Work out the finished part from the listing and answer in its coordinate system (mm). A direction names the side the tool comes from. Coordinates: 2 decimals unless noted, no trailing zeros. Order: outer loops, then holes, each group sorted by start corner. A loop starts at its lowest first (then second) coordinate and runs counter-clockwise, first axis right, second up.
1. The part is cut by section C-C, the plane z = -66. Give the vertices of the cut face in (x, y).
2. Determine the mould class of faces 1 (the flat face through (0.6, -5, -39.8)), 2 (the flat face through (3.133, -3.854, -71.022)) for opening direction Z: +Z half, -Z half, draft (parallel to the pull), parting line (faces both ways), or undercut.
3. The part is cut by section B-B, the plane y = -1.2. Give the vertices of the cut face in (x, z), then the cut area to 3 significant figures.
4. Find the intervals of material crossed by probe 1 along Z at (x, y) = (0, -2.9); probe 2 along X at (y, z) = (-1.6, -16); probe 3 along X at (y, z) = (-2.95, -32), in increasing order.
5. A tool of negligible diameter and unlimited length cuts with its end or side. For faces 3 (the flat face through (3, -2, -40)), 4 (the flat face through (5.61, -2.47, -6.72)), 5 (the flat face through (-4, -1, -40)), 6 (the flat face through (-3.17, -3.48, -10.05)), from which of +Z, -Z, +X, -X, +Y, -Y can it reach the whole face along a straight path? Write none if from no direction.
6. The part is cut by section A-A, the plane z = -55.5. Give the vertices of the cut face in (x, y), then the cut area to 3 significant figures.
7. Flat-ended cylindrical pins translate along their axes: pin 1 Ø0.9 at (y, z) = (-3, -27.5) entering from +X; pin 2 Ø2 at (y, z) = (-3, -68.5) entering from +X; pin 3 Ø1.5 at (y, z) = (-4.5, -25.5) entering from -X. Find the tip coordinate at first contact, or state that the pin passes through.
```python
from build123d import *

# Parameters (mm, degrees)
F0_W      = 4
F0_H      = 5.1029750705
F1_DEPTH  = 5
F4_DEPTH  = 9
F6_W      = 44.082082808
F6_H      = 137.8899626434
F7_DEPTH  = 25
F9_R      = 1.5
F10_DEPTH = 25


with BuildPart() as f1:
    # F0 (on Front) → F1 (new body)
    with BuildSketch(Plane.XZ):
        with Locations((2, -12.5514875352)):
            Rectangle(F0_W, F0_H)
        with BuildLine():
            Line((-4, -10), (0, -10))
            Line((0, -10), (0, -8))
            ThreePointArc((0, -8), (-2.0705523608, -7.7274066103), (-4, -6.9282032303))
            Line((-4, -6.9282032303), (-4, -10))
        make_face()
        with Locations((-2, -12.5514875352)):
            Rectangle(F0_W, F0_H)
        with BuildLine():
            Line((0, -8), (0, -10))
            Line((0, -10), (4, -10))
            Line((4, -10), (4, -6.9282032303))
            ThreePointArc((4, -6.9282032303), (2.0705523608, -7.7274066103), (0, -8))
        make_face()
        with BuildLine():
            Line((4, -15.1029750705), (0, -15.1029750705))
            Line((0, -15.1029750705), (0, -65))
            Line((0, -65), (0, -70))
            Line((0, -70), (0, -72))
            ThreePointArc((0, -72), (2.0705523608, -72.2725933897), (4, -73.0717967697))
            Line((4, -73.0717967697), (4, -70))
            Line((4, -70), (4, -15.1029750705))
        make_face()
        with BuildLine():
            Line((0, -65), (0, -15.1029750705))
            Line((0, -15.1029750705), (-4, -15.1029750705))
            Line((-4, -15.1029750705), (-4, -70))
            Line((-4, -70), (-4, -73.0717967697))
            ThreePointArc((-4, -73.0717967697), (-2.0705523608, -72.2725933897), (0, -72))
            Line((0, -72), (0, -70))
            Line((0, -70), (0, -65))
        make_face()
        with BuildLine():
            ThreePointArc((-4, -6.9282032303), (-2.0705523608, -7.7274066103), (0, -8))
            ThreePointArc((0, -8), (2.0705523608, -7.7274066103), (4, -6.9282032303))
            ThreePointArc((4, -6.9282032303), (5.8428493863, -5.4645320979), (7.1800707248, -3.5279717101))
            ThreePointArc((7.1800707248, -3.5279717101), (7.792322048, -1.8109989235), (8, 0))
            ThreePointArc((8, 0), (-1.8109989235, 7.792322048), (-7.1800707248, -3.5279717101))
            ThreePointArc((-7.1800707248, -3.5279717101), (-5.8428493863, -5.4645320979), (-4, -6.9282032303))
        make_face()
        with BuildLine():
            Line((-7.1800707248, -3.5279717101), (-4, -10))
            Line((-4, -10), (-4, -6.9282032303))
            ThreePointArc((-4, -6.9282032303), (-5.8428493863, -5.4645320979), (-7.1800707248, -3.5279717101))
        make_face()
        with BuildLine():
            Line((4, -6.9282032303), (4, -10))
            Line((4, -10), (7.1800707248, -3.5279717101))
            ThreePointArc((7.1800707248, -3.5279717101), (5.8428493863, -5.4645320979), (4, -6.9282032303))
        make_face()
        with BuildLine():
            Line((-4, -73.0717967697), (-4, -70))
            Line((-4, -70), (-7.1800707248, -76.4720282899))
            ThreePointArc((-7.1800707248, -76.4720282899), (-5.8428493863, -74.5354679021), (-4, -73.0717967697))
        make_face()
        with BuildLine():
            Line((7.1800707248, -76.4720282899), (4, -70))
            Line((4, -70), (4, -73.0717967697))
            ThreePointArc((4, -73.0717967697), (5.8428493863, -74.5354679021), (7.1800707248, -76.4720282899))
        make_face()
        with BuildLine():
            ThreePointArc((4, -73.0717967697), (2.0705523608, -72.2725933897), (0, -72))
            ThreePointArc((0, -72), (-2.0705523608, -72.2725933897), (-4, -73.0717967697))
            ThreePointArc((-4, -73.0717967697), (-5.8428493863, -74.5354679021), (-7.1800707248, -76.4720282899))
            ThreePointArc((-7.1800707248, -76.4720282899), (-1.8109989235, -87.792322048), (8, -80))
            ThreePointArc((8, -80), (7.792322048, -78.1890010765), (7.1800707248, -76.4720282899))
            ThreePointArc((7.1800707248, -76.4720282899), (5.8428493863, -74.5354679021), (4, -73.0717967697))
        make_face()
    extrude(amount=F1_DEPTH)

    # F3 (on offset) → F4 (cut)
    with BuildSketch(Plane.YZ.offset(-10)):
        Polygon((-2, -64.81321129), (-2, -15), (-5.3923702799, -3.64174202), (-5.3923702799, -76.1714303355), align=None)
    extrude(amount=F4_DEPTH, mode=Mode.SUBTRACT)

    # F6 (on Front) → F7 (cut, symmetric)
    with BuildSketch(Plane.XZ):
        with Locations((22.041041404, -24.6477220207)):
            Rectangle(F6_W, F6_H)
    extrude(amount=F7_DEPTH, both=True, mode=Mode.SUBTRACT)

    # F8: F1 across plane


with BuildPart() as f1_1:
    add(f1.part)
    add(f1.part.mirror(Plane.YZ))

    # F9 (on face) → F10 (cut)
    with BuildSketch(Plane.XZ.offset(5)):
        Circle(F9_R)
        with Locations((0, -79.9452960491)):
            Circle(F9_R)
    extrude(amount=-F10_DEPTH, mode=Mode.SUBTRACT)


solid = f1_1.part
```
Geometry says:
1. outline: (-4, -2.35) - (-1, -2.35) - (-1, -5) - (1, -5) - (1, -2.35) - (4, -2.35) - (4, 0) - (-4, 0) - close
2. face 1: draft
2. face 2: undercut
3. outline: (-7.18, -76.47) arc R8 ccw (long way) to (7.18, -76.47) - (4, -70) - (4, -10) - (7.18, -3.53) arc R8 ccw (long way) to (-7.18, -3.53) - (-4, -10) - (-4, -70) - close; hole circle Ø3 at (0, -79.95); hole circle Ø3 at (0, 0)
3. area: 921 mm2
4. probe 1: z = -88 to -81.45, -78.45 to -1.5, 1.5 to 8
4. probe 2: x = -4 to 4
4. probe 3: x = -1 to 1
5. face 3: +X, -Y
5. face 4: +X, +Y, -Y
5. face 5: -X, +Y, -Y
5. face 6: -X, -Y
6. outline: (-4, -2) - (-1, -2) - (-1, -5) - (1, -5) - (1, -2) - (4, -2) - (4, 0) - (-4, 0) - close
6. area: 22.0 mm2
7. pin 1: stops at x = 1
7. pin 2: stops at x = 4
7. pin 3: stops at x = -1
